Autodesk Inventor part; units mm, degrees
ref_plane "YZ Plane" through (0, 0, 0) normal (1, 0, 0) x (0, 1, 0)
ref_plane "XZ Plane" through (0, 0, 0) normal (0, 1, 0) x (-1, 0, 0)
ref_plane "XY Plane" through (0, 0, 0) normal (0, 0, 1) x (1, 0, 0)
sketch "Sketch1" plane through (0, 0, 0) normal (0, 1, 0) x (-1, 0, 0)
  line L0 (-10.795, 10.795) -> (10.795, 10.795)
  line L1 (10.795, 10.795) -> (10.795, -10.795)
  line L2 (-10.795, -10.795) -> (-10.795, 10.795)
  circle A0 centre (5.6576, -5.6576) radius 1.9304
  circle A1 centre (6.9088, 6.9088) radius 1.9304
  circle A2 centre (-5.6576, 5.6576) radius 1.9304
  circle A3 centre (-6.9088, -6.9148) radius 1.9304
  line L3 (-5.715, -10.795) -> (-5.715, -20.574)
  line L4 (-5.715, -20.574) -> (6.985, -20.574)
  line L5 (6.985, -20.574) -> (6.985, -10.795)
  line L6 (10.795, -10.795) -> (6.985, -10.795)
  line L7 (-5.715, -10.795) -> (-10.795, -10.795)
  point P0 (0, 0)
  dimension "d2" = 10.795
  dimension "d3" = 10.795
  dimension "d4" = 3.8608
  dimension "d5" = 5.6576
  dimension "d6" = 5.6576
  dimension "d7" = 3.8608
  dimension "d8" = 6.9088
  dimension "d9" = 6.9088
  dimension "d10" = 3.8608
  dimension "d11" = 5.6576
  dimension "d12" = 5.6576
  dimension "d13" = 3.8608
  dimension "d14" = 12.7
  dimension "d16" = 6.985
  dimension "d45" = 10.795
  dimension "d46" = 10.795
  dimension "d47" = 10.795
extrude "Extrusion1" add sketch "Sketch1" along normal blind 6.985
sketch "Sketch2" plane through (-6.985, 0, -20.574) normal (-1, 0, 0) x (0, 0, 1)
  circle A0 centre (5.08, 3.4925) radius 4.6609 construction
  line L0 (9.779, 0) -> (0, 0)
  line L1 (0, 0) -> (0, 6.985)
  line L2 (9.7409, 3.4925) -> (7.4105, -0.544)
  line L3 (7.4105, -0.544) -> (2.7496, -0.544)
  line L4 (2.7496, -0.544) -> (0.4191, 3.4925)
  line L5 (0.4191, 3.4925) -> (2.7495, 7.529)
  line L6 (2.7495, 7.529) -> (7.4104, 7.529)
  line L7 (7.4104, 7.529) -> (9.7409, 3.4925)
  point P0 (20.574, 0)
  dimension "d19" = 9.3218
  dimension "d20" = 3.4925
  dimension "d21" = 5.08
extrude "Extrusion2" cut sketch "Sketch2" against normal blind 3.81
sketch "Sketch3" plane through (5.715, 0, -10.795) normal (1, 0, 0) x (0, 0, -1)
  circle A0 centre (4.699, 3.4925) radius 1.9304
  line L0 (9.779, 0) -> (9.779, 6.985)
  line L1 (0, 6.985) -> (9.779, 6.985)
  point P0 (-10.795, 0)
  dimension "d24" = 3.8608
  dimension "d25" = 5.08
  dimension "d26" = 3.4925
extrude "Extrusion3" cut sketch "Sketch3" against normal through all
sketch "Sketch4" plane through (0, 6.985, 0) normal (0, 1, 0) x (1, 0, 0)
  circle A0 centre (0, 0) radius 4
  dimension "d29" = 8
extrude "Extrusion4" add sketch "Sketch4" along normal blind 12.7
sketch "Sketch5" plane through (0, 19.685, 0) normal (0, 1, 0) x (1, 0, 0)
  arc A0 (1.8926, -2.4892) -> (-1.8926, -2.4892) centre (0, 0) ccw
  line L0 (-1.8926, -2.4892) -> (1.8926, -2.4892)
  dimension "d32" = 6.254
  dimension "d33" = 2.4892
fillet "Fillet1" radius 3.3782 4 edges at (10.795, 3.4925, 10.795) (10.795, 3.4925, -10.795) (-10.795, 3.4925, 10.795) (-10.795, 3.4925, -10.795)
extrude "Extrusion5" cut sketch "Sketch5" against normal through all
sketch "Sketch6" plane through (0, 19.685, 0) normal (0, 1, 0) x (1, 0, 0)
  line L0 (-6.985, 20.574) -> (5.715, 20.574)
  line L1 (0.635, 0) -> (0.635, 20.574)
  line L2 (0.635, 20.574) -> (-0.635, 20.574)
  line L3 (-0.635, 20.574) -> (-0.635, 0)
  line L4 (-0.635, -20.574) -> (0.635, 20.574) construction
  line L5 (0.635, -20.574) -> (-0.635, 20.574) construction
  line L6 (-0.635, 0) -> (0.635, 0)
  point P0 (0, 0)
  dimension "d37" = 1.27
extrude "Extrusion6" cut sketch "Sketch6" against normal through all
sketch "Sketch7" plane through (0, 0, 0) normal (0, -1, 0) x (1, 0, 0)
  circle A0 centre (-5.6576, -5.6576) radius 1.9304
  circle A1 centre (-5.6576, -5.6576) radius 4.6609 construction
  circle A2 centre (5.6576, 5.6576) radius 1.9304
  circle A3 centre (5.6576, 5.6576) radius 4.6609 construction
  line L0 (-5.6576, -0.9967) -> (-1.6211, -3.3271)
  line L1 (-1.6211, -3.3271) -> (-1.6211, -7.988)
  line L2 (-1.6211, -7.988) -> (-5.6576, -10.3185)
  line L3 (-5.6576, -10.3185) -> (-9.694, -7.988)
  line L4 (-9.694, -7.988) -> (-9.694, -3.3271)
  line L5 (-9.694, -3.3271) -> (-5.6576, -0.9967)
  line L6 (5.6576, 0.9967) -> (1.6211, 3.3271)
  line L7 (1.6211, 3.3271) -> (1.6211, 7.988)
  line L8 (1.6211, 7.988) -> (5.6576, 10.3185)
  line L9 (5.6576, 10.3185) -> (9.694, 7.988)
  line L10 (9.694, 7.988) -> (9.694, 3.3271)
  line L11 (9.694, 3.3271) -> (5.6576, 0.9967)
  point P0 (0, 0)
  dimension "d40" = 9.3218
  dimension "d41" = 9.3218
extrude "Extrusion7" cut sketch "Sketch7" against normal blind 4.3688
fillet "Fillet2" radius 1.27 1 edges at (5.715, 3.4925, -20.574)
properties part number "clamping hub 6mm D"
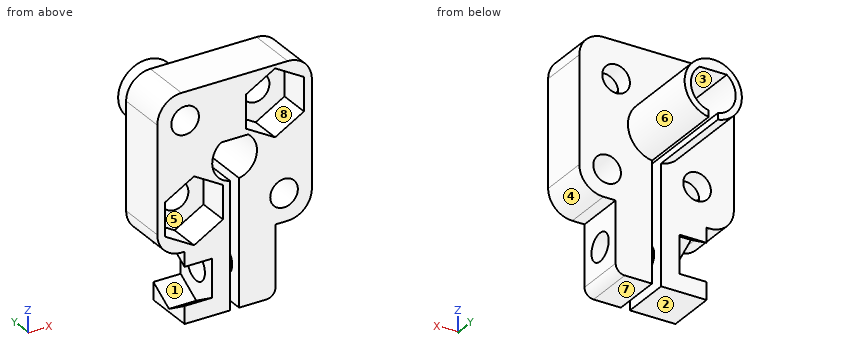
Geometry check sheet. Reference: the model listing, model coordinates, mm. Face numbers are marked on the shaded views. A direction names the side the tool comes from. Give positions to 0.01 mm unless a question says otherwise; leave off trailing zeros. Loops run counter-clockwise (first coordinate to the right, second up) from the corner with the lowest first, then second, coordinate; pieces in that order, holes last. Notation, with made-up numbers: (-18.75, 87) - (26.25, 87) arc R11 ccw to (26.25, 93) - close; hole circle Ø10 at (-20.5, 11.5). An arc over 180 degrees is marked (long way). Use CSV: the item, a comma, the result in double quotes. Start each with the question number.
Q1. Access from +Z, -Z, +X, -X, +Y, -Y to the whole of each face (thin tool, end or side, straight path). Record for the marked faces 1, 2, 3, 4 and 5.
Q2. Release check for a two-part mould opening along Z. For the marked faces 6, 7 and 8 record: +Z half, -Z half, draft (parallel to the pull), parting line (faces both ways), or undercut.
Q3. Go/stop test with flat-tipped pins: pin 1 Ø3 at (x, z) = (-5.5, -13) entering from +Y (3 decimals); pin 2 Ø8 at (x, y) = (-4.5, 12) entering from +Z; pin 3 Ø0.5 at (x, y) = (-7.5, 3) entering from -Z (3 decimals). Record where each tip stops, or that it passes through.
Q4. Section check D-D, the plane x = -4.5. Record the cut outline in (y, z) (1 decimal).
Q5. Section check C-C, the plane y = 16. Record the cut outline in (x, z) (3 decimals).
Q6. Scan lines: probe 1 along X at (y, z) = (2.5, 7) (3 decimals); probe 2 along Z at (x, y) = (2.5, 3) (3 decimals); probe 3 along Z at (x, y) = (-4.25, 4.5) (3 decimals). Record each from-to range of solid material in increasing order. Write a range as from..to.
Q7. Section check A-A, the plane x = 1.25. Record the cut outline in (y, z) (1 decimal).
Q8. Section check B-B, the plane z = 0. Record the cut outline in (x, y) (3 decimals).
Findings below:
1,face 1,"-X"
1,face 2,"-Z, +X, -X, +Y, -Y"
1,face 3,"+Y, -Y"
1,face 4,"-Z, +X, +Y, -Y"
1,face 5,"-Y"
2,face 6,"parting line"
2,face 7,"-Z half"
2,face 8,"undercut"
3,pin 1,"stops at y = 6.985"
3,pin 2,"stops at z = 3.97"
3,pin 3,"stops at z = -10.795"
4,outline,"(0, -20.6) - (7, -20.6) - (7, -18.1) - (3.5, -20.2) - (0, -18.1) - close; (0, -12.8) - (3.5, -10.8) - (7, -12.8) - (7, -7.2) - (4.4, -7.2) - (4.4, -9.7) - (0, -9.7) - close; (0, -1.7) - (4.4, -1.7) - (4.4, -4.1) - (7, -4.1) - (7, 10.8) - (0, 10.8) - close"
5,outline,"(-1.893, 2.489) - (1.893, 2.489) arc R3.127 cw to (0.635, -3.062) - (0.635, -3.949) arc R4 ccw (long way) to (-0.635, -3.949) - (-0.635, -3.062) arc R3.127 cw to start"
6,probe 1,"x = -10.795..-8.837, -4.981..1.621, 9.694..10.795"
6,probe 2,"z = -20.574..-17.361, -13.627..-1.878, 1.878..2.82, 8.495..10.795"
6,probe 3,"z = -20.574..-19.573, -11.415..-6.979, -4.337..10.795"
7,outline,"(0, -20.6) - (7, -20.6) - (7, -3.8) - (19.7, -3.8) - (19.7, -2.9) - (0, -2.9) - close; (0, 2.5) - (19.7, 2.5) - (19.7, 3.8) - (7, 3.8) - (7, 10.8) - (0, 10.8) - close; hole circle Ø3.9 at (3.5, -15.5)"
8,outline,"(-10.795, 0) - (-3.127, 0) - (-3.127, 19.685) - (-4, 19.685) - (-4, 6.985) - (-10.795, 6.985) - close; (3.127, 0) - (10.795, 0) - (10.795, 6.985) - (4, 6.985) - (4, 19.685) - (3.127, 19.685) - close"
